from build123d import *

# Parameters (mm, degrees)
TRAIN_TRACK_DEPTH   = 7.874
TRACK_BASE_SKETCH_W = 1066.8
TRACK_BASE_SKETCH_H = 431.8
TRACK_BASE_DEPTH    = 12.7


with BuildPart() as part:
    # Track Sketch → Train Track (new body)
    with BuildSketch(Plane(origin=(0, 0, 0), x_dir=(1, 0, 0), z_dir=(0, 1, 0))):
        with BuildLine():
            Line((-310, -195.58), (310, -195.58))
            ThreePointArc((310, -195.58), (505.58, 0), (310, 195.58))
            Line((310, 195.58), (-310, 195.58))
            ThreePointArc((-310, 195.58), (-505.58, 0), (-310, -195.58))
        make_face()
        with BuildLine():
            Line((-310, -170.18), (310, -170.18))
            ThreePointArc((310, -170.18), (480.18, 0), (310, 170.18))
            Line((310, 170.18), (-310, 170.18))
            ThreePointArc((-310, 170.18), (-480.18, 0), (-310, -170.18))
        make_face(mode=Mode.SUBTRACT)
    extrude(amount=TRAIN_TRACK_DEPTH)

    # Track Base Sketch → Track Base (add)
    with BuildSketch(Plane(origin=(0, 0, 0), x_dir=(1, 0, 0), z_dir=(0, 1, 0))):
        with Locations((0, -6.35)):
            Rectangle(TRACK_BASE_SKETCH_W, TRACK_BASE_SKETCH_H)
    extrude(amount=-TRACK_BASE_DEPTH)


solid = part.part
Work out the finished part from the listing and answer in its coordinate system (mm). A direction names the side the tool comes from. Give positions to 0.01 mm unless a question says otherwise; leave off trailing zeros. Loops run counter-clockwise (first coordinate to the right, second up) from the corner with the lowest first, then second, coordinate; pieces in that order, holes last. Notation, with made-up numbers: (29, -33.5) -> (35, -33.5) arc R35 cw to (35, 2.5) -> close; hole circle Ø4 at (-0.5, 4.5). An arc over 180 degrees is marked (long way). Use a Markdown table: item, result. Add a question column.
1. Find the intervals of material crossed by probe 1 along Z at (x, y) = (102, 3); probe 2 along Y at (x, z) = (352, 71.5); probe 3 along X at (y, z) = (2.5, -139), in increasing order.
2. Flat-ended cylindrical pins translate along their axes: pin 1 Ø4 at (x, y) = (-26, 5) entering from +Z; pin 2 Ø2.5 at (x, y) = (-132.5, 2.5) entering from -Z. Find the tip coordinate at first contact, or state that the pin passes through.
3. For faces 1 (the cylindrical face through (505.533, 3.882, 4.301)), 2 (the flat face through (-2, 7.874, -175)), 3 (the cylindrical face through (-480.14, 3.88, -3.74)), determine the directions among +Z, -Z, +X, -X, +Y, -Y from which every point of the face is accessible in a straight line to the end or side of a thin tool.
4. Section A-A on y = 4.5 is taken. Determine the outline of the cut face in (x, z), and give its area (3 significant figures).
5. Section B-B on x = 269.5 is taken. Determine the outline of the cut face in (y, z), and give its area (3 significant figures).
6. Section C-C on z = 0 is taken. Determine the outline of the cut face in (x, y), and give its area (3 significant figures).
7. Determine the mould class of faces 4 (the flat face through (-7, 0, -2)), 5 (the cylindrical face through (-505.533, 3.882, -4.301)), 6 (the flat face through (-7, -12.7, 3)) for opening direction X: released by +X, released by -X, zero draft, split by the parting line, or undercut.
Results below:
| question | item | result |
|---|---|---|
| 1 | probe 1 | z = -195.58 to -170.18, 170.18 to 195.58 |
| 1 | probe 2 | y = -12.7 to 0 |
| 1 | probe 3 | x = -447.59 to -408.18, 408.18 to 447.59 |
| 2 | pin 1 | stops at z = 195.58 |
| 2 | pin 2 | stops at z = -195.58 |
| 3 | face 1 | +X, +Y |
| 3 | face 2 | +Z, -Z, +X, -X, +Y |
| 3 | face 3 | +Y |
| 4 | outline | (-310, -195.58) -> (310, -195.58) arc R195.58 ccw to (310, 195.58) -> (-310, 195.58) arc R195.58 ccw to start; hole (-310, -170.18) -> (310, -170.18) arc R170.18 ccw to (310, 170.18) -> (-310, 170.18) arc R170.18 ccw to start |
| 4 | area | 60,700 mm^2 |
| 5 | outline | (-12.7, -209.55) -> (0, -209.55) -> (0, -195.58) -> (7.87, -195.58) -> (7.87, -170.18) -> (0, -170.18) -> (0, 170.18) -> (7.87, 170.18) -> (7.87, 195.58) -> (0, 195.58) -> (0, 222.25) -> (-12.7, 222.25) -> close |
| 5 | area | 5,880 mm^2 |
| 6 | outline | (-533.4, -12.7) -> (533.4, -12.7) -> (533.4, 0) -> (505.58, 0) -> (505.58, 7.87) -> (480.18, 7.87) -> (480.18, 0) -> (-480.18, 0) -> (-480.18, 7.87) -> (-505.58, 7.87) -> (-505.58, 0) -> (-533.4, 0) -> close |
| 6 | area | 13,900 mm^2 |
| 7 | face 4 | undercut |
| 7 | face 5 | released by -X |
| 7 | face 6 | zero draft |
